For this review, take the finished solid that the model builds, in its own axes (mm). Face numbers are marked on the shaded views. A direction names the side the tool comes from. Give positions to 0.01 mm unless a question says otherwise; leave off trailing zeros. Write each loop counter-clockwise with the first axis right and the second up, starting at its lowest first coordinate (ties: lowest second). Pieces come first, ordered by that corner, then holes. Notation, with made-up numbers: M -0.5,61.5 L 52.5,61.5 A26 cw 52.5,78.5 Z; hole C -17.75,-37 d5. An arc over 180 degrees is marked long. Write item = value, one per line.
```python
from build123d import *

# Parameters (mm, degrees)
SKETCH1_R           = 12.5
BOSS_EXTRUDE1_DEPTH = 50
SKETCH2_R           = 3.5
BOSS_EXTRUDE2_DEPTH = 2
SKETCH3_R           = 2
BOSS_EXTRUDE3_DEPTH = 12
SKETCH4_R           = 12.5
SKETCH4_R_2         = 12
CUT_EXTRUDE1_DEPTH  = 30
FILLET1_R           = 1
SKETCH5_R           = 3.070760983
BOSS_EXTRUDE4_DEPTH = 1
FILLET2_R           = 0.5
SKETCH6_R           = 1.5
CUT_EXTRUDE2_DEPTH  = 10


with BuildPart() as part:
    # Sketch1 → Boss-Extrude1 (new body)
    with BuildSketch(Plane.XY):
        Circle(SKETCH1_R)
    extrude(amount=BOSS_EXTRUDE1_DEPTH)

    # Sketch2 → Boss-Extrude2 (add)
    with BuildSketch(Plane.XY.offset(50)):
        Circle(SKETCH2_R)
    extrude(amount=BOSS_EXTRUDE2_DEPTH)

    # Sketch3 → Boss-Extrude3 (add)
    with BuildSketch(Plane.XY.offset(52)):
        Circle(SKETCH3_R)
    extrude(amount=BOSS_EXTRUDE3_DEPTH)

    # Sketch4 → Cut-Extrude1 (cut)
    with BuildSketch(Plane(origin=(0, 0, 0), x_dir=(-1, 0, 0), z_dir=(0, 0, -1))):
        Circle(SKETCH4_R)
        Circle(SKETCH4_R_2, mode=Mode.SUBTRACT)
    extrude(amount=-CUT_EXTRUDE1_DEPTH, mode=Mode.SUBTRACT)

    # Fillet1
    fillet1_edges = [part.edges().sort_by_distance(p)[0] for p in [
        (-12.5, 0, 50),
    ]]
    fillet(fillet1_edges, radius=FILLET1_R)

    # Sketch5 → Boss-Extrude4 (add)
    with BuildSketch(Plane(origin=(0, 0, 0), x_dir=(-1, 0, 0), z_dir=(0, 0, -1))):
        Circle(SKETCH5_R)
    extrude(amount=BOSS_EXTRUDE4_DEPTH)

    # Fillet2
    fillet2_edges = [part.edges().sort_by_distance(p)[0] for p in [
        (3.070760983, 0, -1),
    ]]
    fillet(fillet2_edges, radius=FILLET2_R)

    # Sketch6 → Cut-Extrude2 (cut)
    with BuildSketch(Plane.XY.offset(50)):
        with Locations((8.5, 0)):
            Circle(SKETCH6_R)
        with Locations((-8.5, 0)):
            Circle(SKETCH6_R)
    extrude(amount=-CUT_EXTRUDE2_DEPTH, mode=Mode.SUBTRACT)


solid = part.part
```
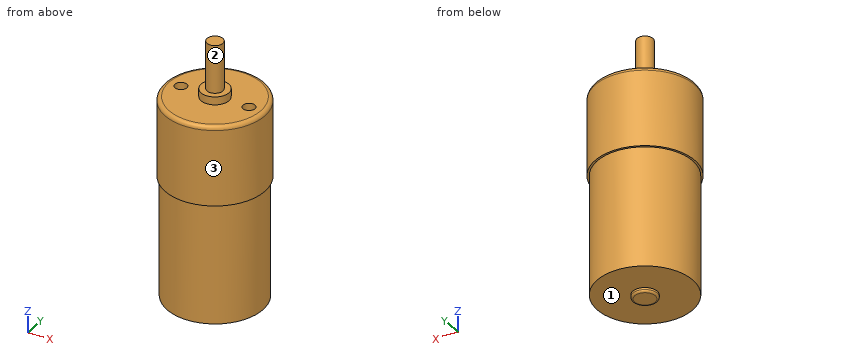
1. Machinability: for the marked faces 1, 2 and 3, which of the approach directions +Z, -Z, +X, -X, +Y, -Y give a long, thin tool a straight path to every point of the face, cutting with its end or side? Answer none if there is none.
Responses:
face_1 = -Z
face_2 = +Z
face_3 = +Z, -Z
2. We need section D-D, the plane z = 33.5. Write out the cut boundary in (x, y), then the cut area to 3 significant figures.
Responses:
outline = C 0,0 d25
area = 491 mm2
3. For line 1 along Z through (x, y) = (3.25, -0.25); line 2 along Y through (x, z) = (-0.5, 47.5); line 3 along Z through (x, y) = (-3.5, 8.25), list the stretches that pass through material, from the lowest coordinate up. Write a range as from..to.
Responses:
line_1 = 0..52
line_2 = -12.49..12.49
line_3 = 0..50
4. Insertion check: P1, Ø10, axis at x = 0, y = 6, coming from the +Z side; P2, Ø2.5, axis at x = -8, y = 0.5, coming from the +Z side; P3, Ø0.9, axis at x = 8, y = 0, coming from the +Z side; P4, Ø1.8, axis at x = 8.5, y = 0, coming from the -Z side. Each pin has a flat end and moves straight along its axis. Give the tip position at first contact, or say it passes through.
Responses:
P1 = 64
P2 = 50
P3 = 40
P4 = 0
5. We need section C-C, the plane z = 24.5. Write out the cut boundary in (x, y).
Responses:
outline = C 0,0 d24
6. We need section B-B, the plane x = 0. Write out the cut boundary in (y, z).
Responses:
outline = M -12.5,30 L -12,30 L -12,0 L -3.07,0 L -3.07,-0.5 A0.5 ccw -2.57,-1 L 2.57,-1 A0.5 ccw 3.07,-0.5 L 3.07,0 L 12,0 L 12,30 L 12.5,30 L 12.5,49 A1 ccw 11.5,50 L 3.5,50 L 3.5,52 L 2,52 L 2,64 L -2,64 L -2,52 L -3.5,52 L -3.5,50 L -11.5,50 A1 ccw -12.5,49 Z
